Check sheet for the modelled part. Datum: model origin and axes. Units: mm. Face numbers are marked on the shaded views. Give positions to 0.01 mm unless a question says otherwise; leave off trailing zeros. Order: outer loops, then holes, each group sorted by start corner. A loop starts at its lowest first (then second) coordinate and runs counter-clockwise, first axis right, second up. Notation, with made-up numbers: (45, 15) -> (93, 15) arc R26 ccw to (93, 32) -> close; hole circle Ø3 at (75.25, 35). An arc over 180 degrees is marked (long way). Answer in a Markdown table with one row per item. Add a question column.
(1) Cross-section at B-B (x = 57.5). Record the cut outline in (y, z).
(2) Cross-section at A-A (x = 31). Record the cut outline in (y, z).
(3) Thickness scan on L1, parallel to X at y = 10.35, z = 5; L2, parallel to X at y = 4.75, z = 4.5; L3, parallel to X at y = 7.95, z = 5. Record the ranges inside material, lowest first. Write a range as [from, to].
(4) Go/stop test with flat-tipped pins: pin 1 (5 mm diameter, centred on x = 62.81, z = 5, fed in from +Y); pin 2 (5 mm diameter, centred on x = 4.81, z = 5, fed in from -Y); pin 3 (2.5 mm diameter, centred on x = 62, z = 4.5, fed in from +Y); pin 4 (1.5 mm diameter, centred on x = 68.5, y = 3, fed in from -Z). Record where each tip stops, or that it passes through.
(5) Release check for a two-part mould opening along X. For the marked faces 1, 2, 3 and 4 record: released by +X, released by -X, zero draft, split by the parting line, or undercut.
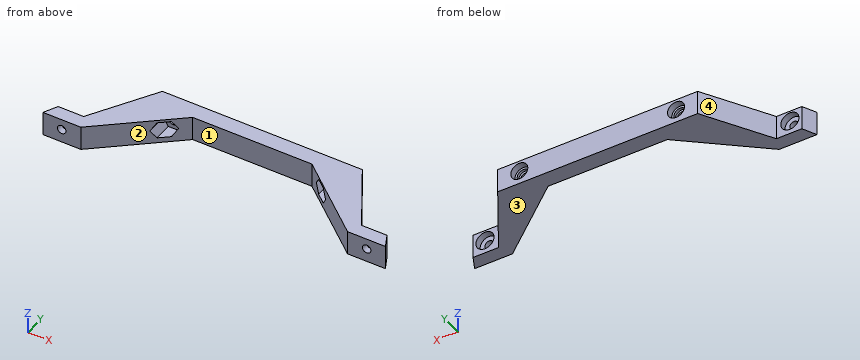
```python
from build123d import *

# Parameters (mm, degrees)
EXTRUDE_1_DEPTH     = 10
SKETCH_7_R          = 1.55
CUT_EXTRUDE_1_DEPTH = 26.214157215
CUT_EXTRUDE_2_DEPTH = 8.5
SKETCH_10_R         = 1.575
CUT_EXTRUDE_4_DEPTH = 12
SKETCH_11_R         = 3.35
CUT_EXTRUDE_5_DEPTH = 2.5
SKETCH_12_W         = 126.714157214
SKETCH_12_H         = 1
CUT_EXTRUDE_6_DEPTH = 29.714157215


with BuildPart() as part:
    # 草图1 → 凸台-拉伸1 (new body)
    with BuildSketch(Plane.XY):
        Polygon((-3.188712924, 13.052848472), (33.811287076, 13.052848472), (33.811287076, 7.052848472), (15.60198174, 7.052848472), (11.74198174, 7.052848472), (-15.549299656, -15.661308743), (-23.688712924, -15.661308743), (-27.545791531, -15.661308743), (-29.545791531, -15.661308743), (-27.045791531, -10.661308743), (-25.045791531, -10.661308743), (-17.614428715, -10.661308743), align=None)
    extrude_1 = extrude(amount=EXTRUDE_1_DEPTH)

    # 镜向1: 凸台-拉伸1 across plane
    add(extrude_1.mirror(Plane(origin=(33.811287076, 13.052848472, 10), x_dir=(0, 0, 1), z_dir=(-1, 0, 0))))

    # 草图5 → 切除-旋转7 (revolve, cut)
    with BuildSketch(Plane.XY.offset(5)):
        Polygon((7.961287076, 13.052848472), (7.961287076, 10.552848472), (7.161287076, 10.552848472), (7.161287076, 9.552848472), (6.361287076, 9.552848472), (4.811287076, 9.552848472), (4.811287076, 13.052848472), align=None)
    cut_revolve_7 = revolve(axis=Axis((4.811287076, 9.552848472, 5), (0, 1, 0)), mode=Mode.SUBTRACT)

    # 草图7 → 切除-拉伸1 (cut, through all)
    with BuildSketch(Plane(origin=(0, 9.552848472, 0), x_dir=(1, 0, 0), z_dir=(0, 1, 0))):
        with Locations((4.811287076, -5)):
            Circle(SKETCH_7_R)
    cut_extrude_1 = extrude(amount=-CUT_EXTRUDE_1_DEPTH, mode=Mode.SUBTRACT)

    # 草图8 → 切除-拉伸2 (cut)
    with BuildSketch(Plane(origin=(0, -1.947151528, 0), x_dir=(1, 0, 0), z_dir=(0, 1, 0))):
        Polygon((8.333123718, -5), (6.572205397, -1.95), (3.050368755, -1.95), (1.289450434, -5), (3.050368755, -8.05), (6.572205397, -8.05), align=None)
    cut_extrude_2 = extrude(amount=CUT_EXTRUDE_2_DEPTH, mode=Mode.SUBTRACT)

    # 草图10 → 切除-拉伸4 (cut)
    with BuildSketch(Plane(origin=(0, -10.661308743, 0), x_dir=(1, 0, 0), z_dir=(0, 1, 0))):
        with Locations((-22.614428715, -5)):
            Circle(SKETCH_10_R)
    cut_extrude_4 = extrude(amount=-CUT_EXTRUDE_4_DEPTH, mode=Mode.SUBTRACT)

    # 草图11 → 切除-拉伸5 (cut)
    with BuildSketch(Plane(origin=(0, -10.661308743, 0), x_dir=(1, 0, 0), z_dir=(0, 1, 0))):
        with Locations((-22.614428715, -5)):
            Circle(SKETCH_11_R)
    cut_extrude_5 = extrude(amount=-CUT_EXTRUDE_5_DEPTH, mode=Mode.SUBTRACT)

    # 镜向2: 切除-旋转7, 切除-拉伸1, 切除-拉伸2, 切除-拉伸4, 切除-拉伸5 across plane
    add(cut_revolve_7.mirror(Plane(origin=(33.811287076, 0, 0), x_dir=(0, 0, 1), z_dir=(1, 0, 0))), mode=Mode.SUBTRACT)
    add(cut_extrude_1.mirror(Plane(origin=(33.811287076, 0, 0), x_dir=(0, 0, 1), z_dir=(1, 0, 0))), mode=Mode.SUBTRACT)
    add(cut_extrude_2.mirror(Plane(origin=(33.811287076, 0, 0), x_dir=(0, 0, 1), z_dir=(1, 0, 0))), mode=Mode.SUBTRACT)
    add(cut_extrude_4.mirror(Plane(origin=(33.811287076, 0, 0), x_dir=(0, 0, 1), z_dir=(1, 0, 0))), mode=Mode.SUBTRACT)
    add(cut_extrude_5.mirror(Plane(origin=(33.811287076, 0, 0), x_dir=(0, 0, 1), z_dir=(1, 0, 0))), mode=Mode.SUBTRACT)

    # 草图12 → 切除-拉伸6 (cut, through all)
    with BuildSketch(Plane(origin=(0, 13.052848472, 0), x_dir=(1, 0, 0), z_dir=(0, 1, 0))):
        with Locations((33.811287076, -9.5)):
            Rectangle(SKETCH_12_W, SKETCH_12_H)
    extrude(amount=-CUT_EXTRUDE_6_DEPTH, mode=Mode.SUBTRACT)


solid = part.part
```
Answer below:
| question | item | result |
|---|---|---|
| 1 | outline | (5.71, 0) -> (13.05, 0) -> (13.05, 9) -> (5.71, 9) -> close |
| 2 | outline | (7.05, 0) -> (13.05, 0) -> (13.05, 9) -> (7.05, 9) -> close |
| 3 | L1 | x = [-4.83, 2.46], [7.16, 60.46], [65.16, 72.46] |
| 3 | L2 | x = [-8.24, 1.58], [8.04, 8.98], [58.65, 59.58], [66.04, 75.86] |
| 3 | L3 | x = [-6.29, 3.26], [6.36, 61.26], [64.36, 73.92] |
| 4 | pin 1 | stops at y = 10.55 |
| 4 | pin 2 | stops at y = 6.55 |
| 4 | pin 3 | stops at y = 9.55 |
| 4 | pin 4 | stops at z = 0 |
| 5 | face 1 | undercut |
| 5 | face 2 | undercut |
| 5 | face 3 | zero draft |
| 5 | face 4 | released by -X |
